```python
from build123d import *

# Parameters (mm, degrees)
F0_W      = 60
F0_H      = 60
F1_DEPTH  = 60
F2_W      = 19
F2_H      = 20
F3_DEPTH  = 60.001
F5_DEPTH  = 60.001
F6_W      = 19
F6_H      = 19
F5_FACE_W = 20
F5_FACE_H = 20
F7_DEPTH  = 25
F9_DEPTH  = 60.001
F11_DEPTH = 20.001
F12_W     = 1
F12_H     = 20
F12_W_2   = 20
F12_H_2   = 1
F13_DEPTH = 2


with BuildPart() as f1:
    # F0 (on Top) → F1 (new body)
    with BuildSketch(Plane.XY):
        Rectangle(F0_W, F0_H)
    extrude(amount=F1_DEPTH)

    # F2 (on face) → F3 (cut, through all)
    with BuildSketch(Plane.XY.offset(60)):
        Polygon((10, -10), (29, -10), (29, 10), (10, 10), (-10, 10), (-10, -29), (10, -29), align=None)
        with Locations((19.5, 20)):
            Rectangle(F2_W, F2_H)
    extrude(amount=-F3_DEPTH, mode=Mode.SUBTRACT)

    # F4 (on face) → F5 (cut, through all)
    with BuildSketch(Plane.XZ.offset(30)):
        Polygon((10, 59), (-10, 59), (-10, 20), (29, 20), (29, 40), (10, 40), align=None)
    extrude(amount=-F5_DEPTH, mode=Mode.SUBTRACT)

    # F6 (on face) + F5_face (on face) → F7 (cut)
    with BuildSketch(Plane.XY.offset(20)):
        with Locations((19.5, -19.5)):
            Rectangle(F6_W, F6_H)
    with BuildSketch(Plane(origin=(18.525, -20.475, 20), x_dir=(1, 0, 0), z_dir=(0, 0, 1))):
        with Locations((-18.525, 40.475)):
            Rectangle(F5_FACE_W, F5_FACE_H)
    extrude(amount=-F7_DEPTH, mode=Mode.SUBTRACT)

    # F8 (on face) → F9 (cut, through all)
    with BuildSketch(Plane.YZ.offset(30)):
        Polygon((-29, 40), (-29, 20), (10, 20), (10, 50), (-10, 50), (-10, 40), align=None)
    extrude(amount=-F9_DEPTH, mode=Mode.SUBTRACT)

    # F10 (on face) → F11 (cut, through all)
    with BuildSketch(Plane.YZ.offset(-10)):
        Polygon((30, 0), (30, 59), (10, 59), (-29, 59), (-29, 40), (-10, 40), (-10, 50), (10, 50), (10, 20), (-29, 20), (-29, 0), align=None)
    extrude(amount=-F11_DEPTH, mode=Mode.SUBTRACT)

    # F12 (on face) → F13 (cut)
    with BuildSketch(Plane.XZ.offset(30)):
        with Locations((29.5, 30)):
            Rectangle(F12_W, F12_H)
        with Locations((0, 59.5)):
            Rectangle(F12_W_2, F12_H_2)
    extrude(amount=-F13_DEPTH, mode=Mode.SUBTRACT)


solid = f1.part
```
Work out the finished part from the listing and answer in its coordinate system (mm). A direction names the side the tool comes from. Give positions to 0.01 mm unless a question says otherwise; leave off trailing zeros. Write each loop counter-clockwise with the first axis right and the second up, starting at its lowest first coordinate (ties: lowest second). Pieces come first, ordered by that corner, then holes.
(1) The part is cut by section C-C on z = 29. Write down the section's boundary in (x, y).
Final values:
outline: (-30, -30) - (-10, -30) - (-10, -29) - (-30, -29) - close; (29, 10) - (30, 10) - (30, 30) - (29, 30) - close
(2) The part is cut by section A-A on y = 7. Write down the section's boundary in (x, z), plus the area to 3 significant figures.
Final values:
outline: (-30, 59) - (-10, 59) - (-10, 60) - (-30, 60) - close; (29, 0) - (30, 0) - (30, 20) - (29, 20) - close; (29, 50) - (30, 50) - (30, 60) - (29, 60) - close
area: 50.0 mm2
(3) Flat-ended cylindrical pins translate along their axes: pin 1 Ø4 at (y, z) = (-23.5, 37) entering from -X; pin 2 Ø3 at (x, y) = (-23, 23.5) entering from -Z; pin 3 Ø0.8 at (x, z) = (-3, 59.5) entering from -Y; pin 4 Ø6 at (x, z) = (21, 52.5) entering from +Y. Find the tip coordinate at first contact, or state that the pin passes through.
Final values:
pin 1: passes through
pin 2: stops at z = 59
pin 3: stops at y = 10
pin 4: stops at y = -10
(4) The mould has two halves that part along X. Classify faces 4 (the flat face through (-10, -29.4, 49)), 5 (the flat face through (-14, -30, 23)), 6 (the flat face through (30, 13, 30)): pulls with the +X half, pulls with the -X half, needs draft (parallel to the pull), parting line crosses it, or undercut.
Final values:
face 4: undercut
face 5: needs draft
face 6: pulls with the +X half
(5) Straight lines are drawn through the part: line 1 (X direction, y = -18.5, z = 10); line 2 (Z direction, x = -9, y = 17); line 3 (Y direction, x = -25.5, z = 6). For each, find the intervals that lie inside material, in ascending order.
Final values:
line 1: x = 29 to 30
line 2: z = 59 to 60
line 3: y = -30 to -29
(6) The part is cut by section D-D on z = 47. Write down the section's boundary in (x, y).
Final values:
outline: (-30, -30) - (-10, -30) - (-10, -29) - (-30, -29) - close; (10, -30) - (30, -30) - (30, -10) - (10, -10) - close; (29, 10) - (30, 10) - (30, 30) - (29, 30) - close
(7) Which of the six approach directions +Z, -Z, +X, -X, +Y, -Y give full straight-line access (tool end or side, diameter ignored) to faces 1 (the flat face through (-14, 7, 59)), 2 (the flat face through (-15, 7, 60)), 3 (the flat face through (18.8, -29.4, 20))?
Final values:
face 1: -Z, -X, +Y
face 2: +Z, +X, -X, +Y, -Y
face 3: +X, -Y
(8) The part is cut by section B-B on x = 2.5. Write down the section's boundary in (y, z), plus the area to 3 significant figures.
Final values:
outline: (-30, 0) - (-29, 0) - (-29, 20) - (-30, 20) - close; (10, 59) - (30, 59) - (30, 60) - (10, 60) - close
area: 40.0 mm2
